Work out the finished part from the listing and answer in its coordinate system (mm). Face numbers are marked on the shaded views. A direction names the side the tool comes from. Coordinates: 2 decimals unless noted, no trailing zeros. One line per item, written item: value.
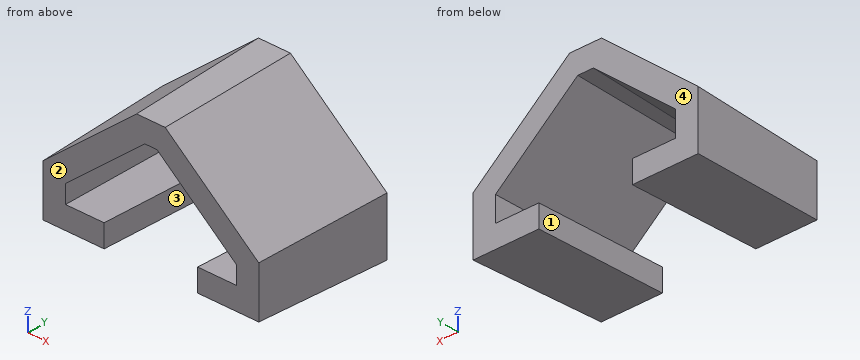
```python
from build123d import *

# Parameters (mm, degrees)
SALIENTE_EXTRUIR1_DEPTH = 75
SALIENTE_EXTRUIR1_TAPER = -2
CORTAR_EXTRUIR1_DEPTH   = 76.0000001
CORTAR_EXTRUIR1_TAPER   = 2
CROQUIS5_W              = 52
CROQUIS5_H              = 12.5
CORTAR_EXTRUIR2_DEPTH   = 76.046325467


with BuildPart() as part:
    # Croquis2 → Saliente-Extruir1 (new body)
    with BuildSketch(Plane(origin=(0, 0, 0), x_dir=(1, 0, 0), z_dir=(0, 1, 0))):
        Polygon((-12.5, 12.5), (-12.5, -15.828845727), (39.545254998, -59.5), (55.454745002, -59.5), (107.5, -15.828845727), (107.5, 12.5), align=None)
    extrude(amount=SALIENTE_EXTRUIR1_DEPTH, taper=SALIENTE_EXTRUIR1_TAPER)

    # Croquis3 → Cortar-Extruir1 (cut, through all)
    with BuildSketch(Plane(origin=(0, 75, 0), x_dir=(1, 0, 0), z_dir=(0, 1, 0))):
        Polygon((-2.619057712, 2.619057712), (-2.619057712, -11.221286668), (43.141623877, -49.619057712), (51.858376123, -49.619057712), (97.619057712, -11.221286668), (97.619057712, 2.619057712), align=None)
    extrude(amount=-CORTAR_EXTRUIR1_DEPTH, taper=CORTAR_EXTRUIR1_TAPER, mode=Mode.SUBTRACT)

    # Croquis5 → Cortar-Extruir2 (cut, through all, along a direction that is not the sketch's normal)
    with BuildSketch(Plane.XZ):
        with Locations((47.5, -6.25)):
            Rectangle(CROQUIS5_W, CROQUIS5_H)
    extrude(amount=-CORTAR_EXTRUIR2_DEPTH, dir=(0, -0.999390827, 0.034899497), mode=Mode.SUBTRACT)


solid = part.part
```
Item 1: Which of the six approach directions +Z, -Z, +X, -X, +Y, -Y give full straight-line access (tool end or side, diameter ignored) to the marked faces 1 and 2?
Evaluation:
face 1: -Z, +Y, -Y
face 2: +Z, -Z, +X, -X, -Y
Item 2: Determine the mould class of the marked faces 3 and 4 for opening direction X: +X half, -X half, draft (parallel to the pull), parting line (faces both ways), or undercut.
Evaluation:
face 3: undercut
face 4: draft
Item 3: Consider probe 1 along X at (y, z) = (61.5, 21); probe 2 along X at (y, z) = (28.5, 4); probe 3 along Z at (x, y) = (75, 47). Determine where each line is inside the solid, lowest interval first.
Evaluation:
probe 1: x = -9.68 to 9.77, 85.23 to 104.68
probe 2: x = -13.5 to -1, 96 to 108.5
probe 3: z = -14.14 to -1.64, 28.92 to 45.24
Item 4: Given pin 1 (1.5 mm diameter, centred on y = 44, z = 36, fed in from +X); pin 2 (2 mm diameter, centred on y = 53, z = 32.5, fed in from -X); pin 3 (2 mm diameter, centred on x = 85, y = 25.5, fed in from +Z), each flat-ended and moving along its own axis, determine where each tip first touches the part or whether it passes through.
Evaluation:
pin 1: stops at x = 86.75
pin 2: stops at x = 3.3
pin 3: stops at z = 36.71
